from build123d import *
from OCP.BRepFilletAPI import BRepFilletAPI_MakeChamfer

# Parameters (mm, degrees)
SKETCH1_R             = 1.95
BOSS_EXTRUDE1_DEPTH   = 9
BOSS_EXTRUDE1_2_DEPTH = 9
BOSS_EXTRUDE2_START   = -3
SKETCH1_3_R           = 1.95
BOSS_EXTRUDE2_DEPTH   = 3
CHAMFER1_SIZE         = 6.08
CHAMFER1_SIZE2        = 0.318639298


with BuildPart() as part:
    # Sketch1 → Boss-Extrude1 (new body)
    with BuildSketch(Plane.XY):
        with Locations((-10, 0)):
            Circle(SKETCH1_R)
    extrude(amount=BOSS_EXTRUDE1_DEPTH)



with BuildPart() as body_2:
    # Sketch1 → Boss-Extrude1 2 (new body)
    with BuildSketch(Plane.XY):
        Circle(SKETCH1_R)
    extrude(amount=BOSS_EXTRUDE1_2_DEPTH)


with BuildPart() as part_1:
    add(part.part)

    add(body_2.part)  # Boss-Extrude2 merges body 2
    # Sketch1_3 → Boss-Extrude2 (add)
    with BuildSketch(Plane.XY.offset(BOSS_EXTRUDE2_START)):
        with BuildLine():
            Line((0, 1.95), (-10, 1.95))
            ThreePointArc((-10, 1.95), (-8.621141777, 1.378858223), (-8.05, 0))
            ThreePointArc((-8.05, 0), (-8.621141777, -1.378858223), (-10, -1.95))
            Line((-10, -1.95), (0, -1.95))
            ThreePointArc((0, -1.95), (-1.95, 0), (0, 1.95))
        make_face()
        with Locations(Location((-10, 0, 0), (0, 0, 90))):
            Circle(SKETCH1_3_R)
        Circle(SKETCH1_3_R)
    extrude(amount=BOSS_EXTRUDE2_DEPTH)

    # Chamfer1: one chamfer whose edges measure the first distance from different faces: ONE call of the kernel's chamfer builder (chamfer() names one face for all edges)
    chamfer1_edges_1 = [part_1.edges().sort_by_distance(p)[0] for p in [
        (-1.95, 0, 9),
    ]]
    chamfer1_side_1 = [part_1.faces().sort_by_distance(p)[0] for p in [
        (-1.378858223, -1.378858223, 3),
    ]]
    chamfer1_edges_2 = [part_1.edges().sort_by_distance(p)[0] for p in [
        (-11.95, 0, 9),
    ]]
    chamfer1_side_2 = [part_1.faces().sort_by_distance(p)[0] for p in [
        (-11.95, 0, 3),
    ]]
    chamfer1 = BRepFilletAPI_MakeChamfer(part_1.part.solid().wrapped)
    for e in chamfer1_edges_1:
        chamfer1.Add(CHAMFER1_SIZE, CHAMFER1_SIZE2, e.wrapped, chamfer1_side_1[0].wrapped)  # the first distance lies on this face
    for e in chamfer1_edges_2:
        chamfer1.Add(CHAMFER1_SIZE, CHAMFER1_SIZE2, e.wrapped, chamfer1_side_2[0].wrapped)  # the first distance lies on this face
    add(Compound.cast(chamfer1.Shape()), mode=Mode.REPLACE)


solid = part_1.part
Model file for the job. Use its own axes, mm. A direction names the side the tool comes from. Give positions to 0.01 mm unless a question says otherwise; leave off trailing zeros. Order: outer loops, then holes, each group sorted by start corner. A loop starts at its lowest first (then second) coordinate and runs counter-clockwise, first axis right, second up. Notation, with made-up numbers: (13, 8) -> (28, 8) arc R12 cw to (28, 30) -> close; hole circle Ø5 at (-31.75, 52). An arc over 180 degrees is marked (long way). Use CSV: the item, a comma, the result in double quotes.
1. Band-saw the part on D-D, the plane z = -1.75. Give the cut face in (x, y), then the cut area to 3 significant figures.
Outcome:
outline,"(-10, -1.95) -> (0, -1.95) arc R1.95 ccw to (0, 1.95) -> (-10, 1.95) arc R1.95 ccw to start"
area,"50.9 mm²"
2. Band-saw the part on C-C, the plane x = -6. Give the cut face in (y, z).
Outcome:
outline,"(-1.95, -3) -> (1.95, -3) -> (1.95, 0) -> (-1.95, 0) -> close"
3. Mould opens along X. For faces 1 (the flat face through (-10, 0, 9)), 2 (the conical face through (-1.42, -1.09, 6)) say: +X half, -X half, draft (parallel to the pull), parting line (faces both ways), or undercut.
Outcome:
face 1,"draft"
face 2,"undercut"
4. Band-saw the part on A-A, the plane z = 2. Give the cut face in (x, y).
Outcome:
outline,"circle Ø3.9 at (-10, 0); circle Ø3.9 at (0, 0)"
5. Drop a flat-ended pin along its axis: pin 1 (1.2 mm diameter, centred on x = -7, y = 0, fed in from +Z). Give the stop position or say it passes through.
Outcome:
pin 1,"z = 0"
6. Drill centre lines: line 1 along X through (y, z) = (-0.65, 5); line 2 along X through (y, z) = (-0.3, 3.25); line 3 along Z through (x, y) = (-6.75, 0.25). Where is each one in solid material? Low to high. Write a range as from..to.
Outcome:
line 1,"-11.72..-8.28, -1.72..1.72"
line 2,"-11.91..-8.09, -1.91..1.91"
line 3,"-3..0"
7. Band-saw the part on B-B, the plane y = 0. Give the cut face in (x, z), then the cut area to 3 significant figures.
Outcome:
outline,"(-11.95, -3) -> (1.95, -3) -> (1.95, 2.92) -> (1.63, 9) -> (-1.63, 9) -> (-1.95, 2.92) -> (-1.95, 0) -> (-8.05, 0) -> (-8.05, 2.92) -> (-8.37, 9) -> (-11.63, 9) -> (-11.95, 2.92) -> close"
area,"108 mm²"
8. 3-axis set-ups, long thin cutter, end or side, ignore diameter. For faces 3 (the cylindrical face through (1.72, -0.92, -0.08)), 4 (the flat face through (-5, 1.95, -2)): which of +Z, -Z, +X, -X, +Y, -Y reach the whole face in a straight line?
Outcome:
face 3,"+Z"
face 4,"+Z, -Z, +X, -X, +Y"
